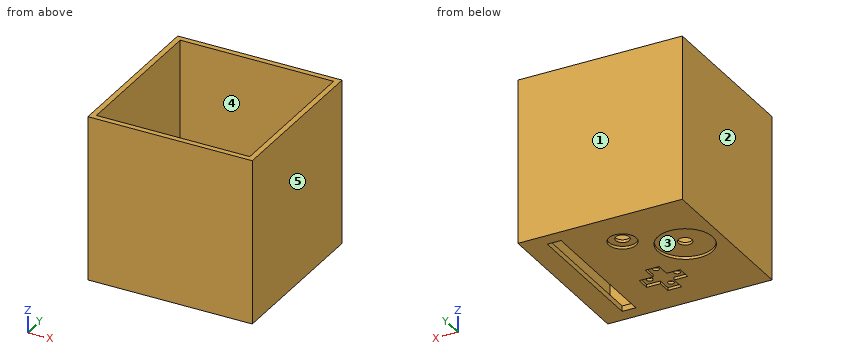
from build123d import *

# Parameters (mm, degrees)
SKETCH1_W               = 76.2
SKETCH1_H               = 76.2
BOX_DEPTH               = 76.2
HOLLOW_IT_T             = -2.54
SKETCH2_W               = 6.35
SKETCH2_H               = 63.5
SLIDER_TRACK_DEPTH      = 2.54
SKETCH4_R               = 6.35
BUTTON_LARGE_RING_DEPTH = 1.27
SKETCH5_R               = 3.175
BUTTON_SMALL_HOLE_DEPTH = 1.27
DPAD_LARGE_SHAPE_DEPTH  = 1.27
SKETCH7_R               = 1.397
DPAD_TINY_HOLES_DEPTH   = 1.27
SKETCH8_R               = 12.7
DIAL_LARGE_RING_DEPTH   = 1.27
SKETCH9_R               = 3.175
DIAL_SMALL_HOLE_DEPTH   = 1.27


with BuildPart() as part:
    # Sketch1 → box (new body)
    with BuildSketch(Plane(origin=(0, 0, 0), x_dir=(1, 0, 0), z_dir=(0, 1, 0))):
        Rectangle(SKETCH1_W, SKETCH1_H)
    extrude(amount=BOX_DEPTH)

    # hollow it
    hollow_it_openings = [part.faces().sort_by_distance(p)[0] for p in [
        (0, 38.1, 38.1),
    ]]
    offset(amount=HOLLOW_IT_T, openings=hollow_it_openings, kind=Kind.INTERSECTION)

    # Sketch2 → slider track (cut)
    with BuildSketch(Plane(origin=(0, 0, -38.1), x_dir=(-1, 0, 0), z_dir=(0, 0, -1))):
        with Locations((-24.765, 38.1)):
            Rectangle(SKETCH2_W, SKETCH2_H)
    extrude(amount=-SLIDER_TRACK_DEPTH, mode=Mode.SUBTRACT)

    # Sketch4 → button large ring (cut)
    with BuildSketch(Plane(origin=(0, 0, -38.1), x_dir=(-1, 0, 0), z_dir=(0, 0, -1))):
        with Locations((0, 57.15)):
            Circle(SKETCH4_R)
    extrude(amount=-BUTTON_LARGE_RING_DEPTH, mode=Mode.SUBTRACT)

    # Sketch5 → button small hole (cut)
    with BuildSketch(Plane(origin=(0, 0, -36.83), x_dir=(-1, 0, 0), z_dir=(0, 0, -1))):
        with Locations((0, 57.15)):
            Circle(SKETCH5_R)
    extrude(amount=-BUTTON_SMALL_HOLE_DEPTH, mode=Mode.SUBTRACT)

    # Sketch6 → dpad large shape (cut)
    with BuildSketch(Plane(origin=(0, 0, -38.1), x_dir=(-1, 0, 0), z_dir=(0, 0, -1))):
        Polygon((-3.297705804, 25.4), (-3.297705804, 31.75), (3.052294196, 31.75), (3.052294196, 25.4), (9.402294196, 25.4), (9.402294196, 19.05), (3.052294196, 19.05), (3.052294196, 12.7), (-3.297705804, 12.7), (-3.297705804, 19.05), (-9.647705804, 19.05), (-9.647705804, 25.4), align=None)
    extrude(amount=-DPAD_LARGE_SHAPE_DEPTH, mode=Mode.SUBTRACT)

    # Sketch7 → dpad tiny holes (cut)
    with BuildSketch(Plane(origin=(0, 0, -36.83), x_dir=(-1, 0, 0), z_dir=(0, 0, -1))):
        with Locations((-0.122705804, 28.575)):
            Circle(SKETCH7_R)
        with Locations((6.227294196, 22.225)):
            Circle(SKETCH7_R)
        with Locations((-0.122705804, 15.875)):
            Circle(SKETCH7_R)
        with Locations((-6.472705804, 22.225)):
            Circle(SKETCH7_R)
    extrude(amount=-DPAD_TINY_HOLES_DEPTH, mode=Mode.SUBTRACT)

    # Sketch8 → dial large ring (cut)
    with BuildSketch(Plane(origin=(0, 0, -38.1), x_dir=(-1, 0, 0), z_dir=(0, 0, -1))):
        with Locations((21.336, 43.050678032)):
            Circle(SKETCH8_R)
    extrude(amount=-DIAL_LARGE_RING_DEPTH, mode=Mode.SUBTRACT)

    # Sketch9 → dial small hole (cut)
    with BuildSketch(Plane(origin=(0, 0, -36.83), x_dir=(-1, 0, 0), z_dir=(0, 0, -1))):
        with Locations((21.336, 43.050678032)):
            Circle(SKETCH9_R)
    extrude(amount=-DIAL_SMALL_HOLE_DEPTH, mode=Mode.SUBTRACT)


solid = part.part
Verification items for the finished model (mm, model axes). Face numbers are marked on the shaded views. A direction names the side the tool comes from. Give positions to 0.01 mm unless a question says otherwise; leave off trailing zeros. Loops run counter-clockwise (first coordinate to the right, second up) from the corner with the lowest first, then second, coordinate; pieces in that order, holes last.
1) Draft check along X on the marked faces 1, 2 and 3. Enter one of: pulls with the +X half, pulls with the -X half, needs draft (parallel to the pull), parting line crosses it, or undercut.
2) Sectioned sample at D-D, the plane y = 57.15. Enter the section's corners in (x, z) (3 decimals).
3) Sectioned sample at C-C, the plane x = 0. Enter the section's corners in (y, z) (3 decimals).
4) Set-up check for the marked faces 4 and 5: record each of +Z, -Z, +X, -X, +Y, -Y from which the full face is reachable in a straight line by a thin tool's end or side.
5) Depth check by flat-ended pin: pin 1 Ø3.5 at (x, y) = (-6.23, 22.22) entering from -Z; pin 2 Ø4 at (x, y) = (0, 57.15) entering from -Z. Enter the tip coordinate at first touch or a pass-through.
6) Sectioned sample at B-B, the plane y = 8. Enter the section's corners in (x, z), then the cut area to 3 significant figures.
7) Thickness scan on line 1 along Y through (x, z) = (0, -37.1); line 2 along Y through (x, z) = (-1.5, -17); line 3 along X through (y, z) = (55, 26). Record the ranges inside material, lowest first.
8) Sectioned sample at A-A, the plane z = 30. Enter the section's corners in (x, y).
Answers:
1. face 1: needs draft
1. face 2: pulls with the -X half
1. face 3: undercut
2. outline: (-38.1, -38.1) - (-6.35, -38.1) - (-6.35, -36.83) - (-3.175, -36.83) - (-3.175, -35.56) - (-35.56, -35.56) - (-35.56, 38.1) - (-38.1, 38.1) - close; (3.175, -36.83) - (6.35, -36.83) - (6.35, -38.1) - (21.59, -38.1) - (21.59, -35.56) - (3.175, -35.56) - close; (27.94, -38.1) - (38.1, -38.1) - (38.1, 38.1) - (35.56, 38.1) - (35.56, -35.56) - (27.94, -35.56) - close
3. outline: (0, -38.1) - (12.7, -38.1) - (12.7, -36.83) - (14.483, -36.83) - (14.483, -35.56) - (2.54, -35.56) - (2.54, 38.1) - (0, 38.1) - close; (17.267, -36.83) - (27.183, -36.83) - (27.183, -35.56) - (17.267, -35.56) - close; (29.967, -36.83) - (31.75, -36.83) - (31.75, -38.1) - (50.8, -38.1) - (50.8, -36.83) - (53.975, -36.83) - (53.975, -35.56) - (29.967, -35.56) - close; (60.325, -36.83) - (63.5, -36.83) - (63.5, -38.1) - (76.2, -38.1) - (76.2, 38.1) - (73.66, 38.1) - (73.66, -35.56) - (60.325, -35.56) - close
4. face 4: +Z
4. face 5: +Z, -Z, +X, +Y, -Y
5. pin 1: stops at z = -36.83
5. pin 2: passes through
6. outline: (-38.1, -38.1) - (21.59, -38.1) - (21.59, -35.56) - (-35.56, -35.56) - (-35.56, 38.1) - (-38.1, 38.1) - close; (27.94, -38.1) - (38.1, -38.1) - (38.1, 38.1) - (35.56, 38.1) - (35.56, -35.56) - (27.94, -35.56) - close
6. area: 552 mm2
7. line 1: y = 0 to 12.7, 31.75 to 50.8, 63.5 to 76.2
7. line 2: y = 0 to 2.54, 73.66 to 76.2
7. line 3: x = -38.1 to -35.56, 35.56 to 38.1
8. outline: (-38.1, 0) - (38.1, 0) - (38.1, 76.2) - (-38.1, 76.2) - close; hole (-35.56, 2.54) - (35.56, 2.54) - (35.56, 73.66) - (-35.56, 73.66) - close
